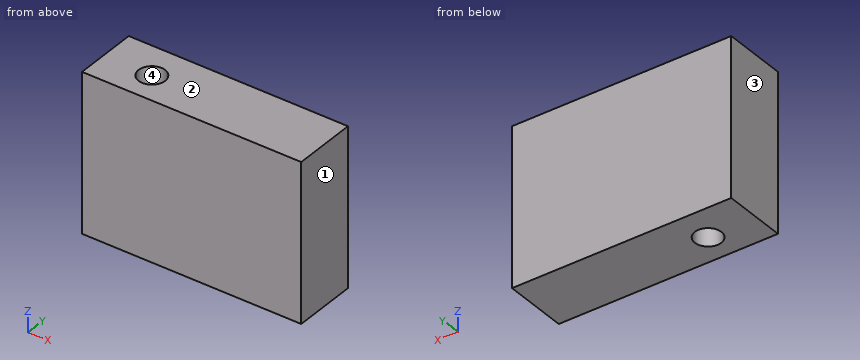
from build123d import *

# Parameters (mm, degrees)
F0_W     = 41.2274915725
F0_H     = 29.704278335
F2_DEPTH = 12
F5_D     = 5


# Not quite as in the source:
# - the program builds the solid bodies; features that only make, move or delete a surface that nothing else refers to are left out


with BuildPart() as f2:
    # F0 (on Front) → F2 (new body)
    with BuildSketch(Plane.XZ):
        with Locations((0.2560736611, -0.512146391)):
            Rectangle(F0_W, F0_H)
    extrude(amount=F2_DEPTH)

    # F5 (through all)
    with Locations(Plane.XY.offset(14.3399927765)):
        with Locations((-11.2421652302, -6.5094744787)):
            Hole(F5_D / 2)


solid = f2.part
Geometry check sheet. Reference: the model listing, model coordinates, mm. Face numbers are marked on the shaded views. Give positions to 0.01 mm unless a question says otherwise; leave off trailing zeros. Order: outer loops, then holes, each group sorted by start corner. A loop starts at its lowest first (then second) coordinate and runs counter-clockwise, first axis right, second up. Notation, with made-up numbers: M 1.25,83.25 L 23.25,83.25 A29 cw 23.25,121.25 Z; hole C 2,-10.5 d11. An arc over 180 degrees is marked long. Use a Markdown table: item, result.
Item 1: Draft check along X on the marked faces 1, 2, 3 and 4. Enter one of: +X half, -X half, draft (parallel to the pull), parting line (faces both ways), or undercut.
Answers follow:
| item | result |
|---|---|
| face 1 | +X half |
| face 2 | draft |
| face 3 | -X half |
| face 4 | undercut |
Item 2: Section check B-B (z = 10.75). Record the cut outline in (x, y).
Answers follow:
| item | result |
|---|---|
| outline | M -20.36,-12 L 20.87,-12 L 20.87,0 L -20.36,0 Z; hole C -11.24,-6.51 d5 |
Item 3: Section check A-A (y = -5.75). Record the cut outline in (x, z).
Answers follow:
| item | result |
|---|---|
| outline | M -20.36,-15.36 L -13.62,-15.36 L -13.62,14.34 L -20.36,14.34 Z; M -8.86,-15.36 L 20.87,-15.36 L 20.87,14.34 L -8.86,14.34 Z |
Item 4: Material ranges on line 1 along X through (y, z) = (-6.5, -12.75); line 2 along X through (y, z) = (-5, -5.75); line 3 along Y through (x, z) = (-9, -7), recorded low to high.
Answers follow:
| item | result |
|---|---|
| line 1 | x = -20.36 to -13.74, -8.74 to 20.87 |
| line 2 | x = -20.36 to -13.24, -9.25 to 20.87 |
| line 3 | y = -12 to -7.62, -5.4 to 0 |
